Build history of the part. All positions in model axes, mm. A direction names the side the tool comes from. Round coordinates to 2 decimals unless told otherwise and drop trailing zeros. Order: outer loops, then holes, each group sorted by start corner. A loop starts at its lowest first (then second) coordinate and runs counter-clockwise, first axis right, second up. Notation, with made-up numbers: M 26.25,9 L 54.25,9 A19 ccw 54.25,25 Z; hole C 14,47.5 d7. An arc over 180 degrees is marked long. One line per item, written item: value. Start each with the question number.
Item 1: Tool access for faces 5 (the cylindrical face through (18.73, -0.15, 21.46)), 6 (the flat face through (0, 2, 21)), 7 (the flat face through (-2, -2, 21)): list every direction of +Z, -Z, +X, -X, +Y, -Y with a clear straight run to the whole face (end or side of a thin tool).
Item 2: Pin check, flat tips, straight feed: pin 1 (2.5 mm diameter, centred on x = 20.5, y = -0.5, fed in from -Z); pin 2 (3 mm diameter, centred on y = 0.5, z = 37, fed in from +X); pin 3 (10.5 mm diameter, centred on x = -6.5, z = 28, fed in from -Y); pin 4 (3.5 mm diameter, centred on x = -11.82, z = 11.5, fed in from -Y). Stop position of each tip, or through.
Item 3: Probe L1, parallel to Z at x = 23, y = -5.5; L2, parallel to Y at x = -9.5, z = 29; L3, parallel to X at y = -2.75, z = 15. List the from-to ranges inside material, lowest first.
Item 4: Two-plate mould, pull along Y, no slides. Class faces 1 (the flat face through (-1, 0, 43)), 2 (the flat face through (17.512, -2.845, 21.199)), 3 (the cylindrical face through (18.73, -0.15, 40.52)), 4 (the cylindrical face through (18.73, -0.15, 2.46)): +Y half, -Y half, draft (parallel to the pull), parting line (faces both ways), or undercut.
Item 5: Band-saw the part on C-C, the plane y = 0.25. Write the cut outline in (x, z).
Item 6: Band-saw the part on B-B, the plane y = -4.25. Write the cut outline in (x, z).
Item 7: Band-saw the part on A-A, the plane z = 11.5. Write the cut outline in (x, y).
Item 8: Band-saw the part on D-D, the plane x = -16.5. Write the cut outline in (y, z).
```python
from build123d import *

# Parameters (mm, degrees)
F1_DEPTH    = 43
F2_T1_DEPTH = 43
F2_T3_DEPTH = 58.4300979278
F4_D        = 4.4
F5_R        = 4.2
F6_DEPTH    = 5
F7_START    = 15.1
F7_DEPTH    = 12.9
F8_START    = 38.1
F8_DEPTH    = 11.9


# Not quite as in the source:
# - a fillet or chamfer that OpenCascade refuses, or shapes differently, is made with other operations: its cross-section is extruded or revolved along the edge and cut away or added


with BuildPart() as f1:
    # F0 (on Top) → F1 (new body)
    with BuildSketch(Plane.XY):
        with BuildLine():
            Line((-22.5, -2), (18.5, -2))
            ThreePointArc((18.5, -2), (19.6715728753, 0.8284271247), (22.5, 2))
            Line((22.5, 2), (-22.5, 2))
            Line((-22.5, 2), (-22.5, -2))
        make_face()
        with BuildLine():
            Line((18.5, -2), (21.4, -2))
            ThreePointArc((21.4, -2), (21.7221825407, -1.2221825407), (22.5, -0.9))
            Line((22.5, -0.9), (22.5, 2))
            ThreePointArc((22.5, 2), (19.6715728753, 0.8284271247), (18.5, -2))
        make_face()
        with BuildLine():
            ThreePointArc((23.6, -2), (22.5, -3.1), (21.4, -2))
            Line((21.4, -2), (18.5, -2))
            ThreePointArc((18.5, -2), (22.5, -6), (26.5, -2))
            ThreePointArc((26.5, -2), (25.3284271247, 0.8284271247), (22.5, 2))
            Line((22.5, 2), (22.5, -0.9))
            ThreePointArc((22.5, -0.9), (23.2778174593, -1.2221825407), (23.6, -2))
        make_face()
    extrude(amount=F1_DEPTH)

    # F2: chamfer of 3 on 2 edges, made by hand

    # F2_s2 → F2_t1 (join)
    with BuildSketch(Plane.XY):
        with BuildLine():
            Line((16.0740261691, -1.9358573019), (18.9873868989, -3.7784284123))
            Line((18.9873868989, -3.7784284123), (19.0415973731, -3.7527141266))
            ThreePointArc((19.0415973731, -3.7527141266), (18.6659635809, -2.9076148618), (18.56, -2))
            Line((18.56, -2), (18.5, -1.94))
            ThreePointArc((18.5, -1.94), (17.2870130845, -1.94), (16.0740261691, -1.8758573019))
            Line((16.0740261691, -1.8758573019), (16.0740261691, -1.9358573019))
        make_face()
    extrude(amount=F2_T1_DEPTH)

    # F2_s4 → F2_t3 (cut)
    with BuildSketch(Plane.XY.offset(-7.7150489639)):
        with BuildLine():
            Line((-22.5848528137, 1.0848528137), (-19.4151471863, -2.0848528137))
            Line((-19.4151471863, -2.0848528137), (-19.4151471863, -2.1448528137))
            ThreePointArc((-19.4151471863, -2.1448528137), (-20.9575735931, -2.06), (-22.5, -2.06))
            Line((-22.5, -2.06), (-22.56, -2))
            ThreePointArc((-22.56, -2), (-22.56, -0.4575735931), (-22.6448528137, 1.0848528137))
            Line((-22.6448528137, 1.0848528137), (-22.5848528137, 1.0848528137))
        make_face()
    extrude(amount=F2_T3_DEPTH, mode=Mode.SUBTRACT)

    # F4 (through all)
    with Locations(Plane.XZ.offset(2)):
        with Locations((-11.8245553203, 31.5), (-11.8245553203, 11.5)):
            Hole(F4_D / 2)

    # F5 (on face) → F6 (cut)
    with BuildSketch(Plane.XY):
        with Locations((22.5, -2)):
            Circle(F5_R)
    extrude(amount=F6_DEPTH, mode=Mode.SUBTRACT)

    # F5 (on face) → F7 (cut)
    with BuildSketch(Plane.XY.offset(F7_START)):
        with Locations((22.5, -2)):
            Circle(F5_R)
    extrude(amount=F7_DEPTH, mode=Mode.SUBTRACT)

    # F5 (on face) → F8 (cut)
    with BuildSketch(Plane.XY.offset(F8_START)):
        with Locations((22.5, -2)):
            Circle(F5_R)
    extrude(amount=F8_DEPTH, mode=Mode.SUBTRACT)


solid = f1.part
```
Output:
1. face 5: +X
1. face 6: +Z, -Z, +X, -X, +Y
1. face 7: +Z, -Z, -X, -Y
2. pin 1: stops at z = 5
2. pin 2: stops at x = 26.37
2. pin 3: stops at y = -2
2. pin 4: passes through
3. L1: z = 5 to 15.1, 28 to 38.1
3. L2: y = -2 to 2
3. L3: x = 17.36 to 21.7, 23.3 to 26.43
4. face 1: draft
4. face 2: -Y half
4. face 3: undercut
4. face 4: undercut
5. outline: M -21.75,0 L 18.95,0 L 18.95,5 L 25.81,5 L 25.81,15.1 L 18.95,15.1 L 18.95,28 L 25.81,28 L 25.81,38.1 L 18.95,38.1 L 18.95,43 L -21.75,43 Z; hole C -11.82,11.5 d4.4; hole C -11.82,31.5 d4.4
6. outline: M 19.19,5 L 25.81,5 L 25.81,15.1 L 19.19,15.1 Z; M 19.19,28 L 25.81,28 L 25.81,38.1 L 19.19,38.1 Z
7. outline: M -22.5,1 L -19.5,-2 L -14.02,-2 L -14.02,2 L -22.5,2 Z; M -9.62,-2 L 16.18,-2 L 18.89,-3.71 A4 ccw long 22.5,2 L -9.62,2 Z; hole C 22.5,-2 d2.2
8. outline: M -2,0 L 2,0 L 2,43 L -2,43 Z
